Geometry: final body of the model. Coordinates: model frame, mm. Give positions to 0.01 mm unless a question says otherwise; leave off trailing zeros. Write each loop counter-clockwise with the first axis right and the second up, starting at its lowest first coordinate (ties: lowest second). Pieces come first, ordered by that corner, then holes. Notation, with made-up numbers: M 45,-33 L 54,-33 A17 cw 54,-13 Z; hole C -14,87.5 d6. An arc over 180 degrees is marked long. Answer as a JSON object with one key per item and string values.
Autodesk Fusion 360 part; units mm, degrees
sketch "plate-2025-12-04T13_16_58.583Z" plane through (0, 0, 0) normal (0, 0, 1) x (1, 0, 0)
  line L0 (3.025, -21.575) -> (16.025, -21.575)
  line L1 (3.025, -35.575) -> (16.025, -35.575)
  line L2 (2.525, -22.075) -> (2.525, -35.075)
  line L3 (16.525, -22.075) -> (16.525, -35.075)
  arc A0 (3.025, -21.575) -> (2.525, -22.075) centre (3.025, -22.075) ccw
  arc A1 (16.525, -22.075) -> (16.025, -21.575) centre (16.025, -22.075) ccw
  arc A2 (2.525, -35.075) -> (3.025, -35.575) centre (3.025, -35.075) ccw
  arc A3 (16.025, -35.575) -> (16.525, -35.075) centre (16.025, -35.075) ccw
  line L4 (22.075, -21.575) -> (35.075, -21.575)
  line L5 (22.075, -35.575) -> (35.075, -35.575)
  line L6 (21.575, -22.075) -> (21.575, -35.075)
  line L7 (35.575, -22.075) -> (35.575, -35.075)
  arc A4 (22.075, -21.575) -> (21.575, -22.075) centre (22.075, -22.075) ccw
  arc A5 (35.575, -22.075) -> (35.075, -21.575) centre (35.075, -22.075) ccw
  arc A6 (21.575, -35.075) -> (22.075, -35.575) centre (22.075, -35.075) ccw
  arc A7 (35.075, -35.575) -> (35.575, -35.075) centre (35.075, -35.075) ccw
  line L8 (3.025, -40.625) -> (16.025, -40.625)
  line L9 (3.025, -54.625) -> (16.025, -54.625)
  line L10 (2.525, -41.125) -> (2.525, -54.125)
  line L11 (16.525, -41.125) -> (16.525, -54.125)
  arc A8 (3.025, -40.625) -> (2.525, -41.125) centre (3.025, -41.125) ccw
  arc A9 (16.525, -41.125) -> (16.025, -40.625) centre (16.025, -41.125) ccw
  arc A10 (2.525, -54.125) -> (3.025, -54.625) centre (3.025, -54.125) ccw
  arc A11 (16.025, -54.625) -> (16.525, -54.125) centre (16.025, -54.125) ccw
  line L12 (22.075, -40.625) -> (35.075, -40.625)
  line L13 (22.075, -54.625) -> (35.075, -54.625)
  line L14 (21.575, -41.125) -> (21.575, -54.125)
  line L15 (35.575, -41.125) -> (35.575, -54.125)
  arc A12 (22.075, -40.625) -> (21.575, -41.125) centre (22.075, -41.125) ccw
  arc A13 (35.575, -41.125) -> (35.075, -40.625) centre (35.075, -41.125) ccw
  arc A14 (21.575, -54.125) -> (22.075, -54.625) centre (22.075, -54.125) ccw
  arc A15 (35.075, -54.625) -> (35.575, -54.125) centre (35.075, -54.125) ccw
  line L16 (0, -57.15) -> (38.1, -57.15)
  line L17 (0, -19.05) -> (38.1, -19.05)
  line L18 (0, -57.15) -> (0, -19.05)
  line L19 (38.1, -57.15) -> (38.1, -19.05)
  line L20 (-17.994, 26.134) -> (60.006, 26.134)
  line L21 (60.006, 26.134) -> (60.006, -68.197)
  line L22 (60.006, -68.197) -> (-17.994, -68.197)
  line L23 (-17.994, -68.197) -> (-17.994, 26.134)
  line L24 (6.604, 26.134) -> (25.104, 26.134)
  line L25 (25.104, 26.134) -> (25.104, -4.866)
  line L26 (25.104, -4.866) -> (6.604, -4.866)
  line L27 (6.604, -4.866) -> (6.604, 26.134)
  circle A16 centre (-12.994, 21.134) radius 1.7
  circle A17 centre (55.006, 21.134) radius 1.7
  circle A18 centre (-12.994, -63.197) radius 1.7
  circle A19 centre (55.006, -63.197) radius 1.7
  dimension "d1" = 78
  dimension "d2" = 94.331
  dimension "d4" = 20.519
  dimension "d5" = 13.572
  dimension "d6" = 18.5
  dimension "d7" = 31
  dimension "d8" = 24.598
  dimension "d9" = 3.4
  dimension "d10" = 5
  dimension "d11" = 5
  dimension "d12" = 3.4
  dimension "d13" = 5
  dimension "d14" = 5
  dimension "d15" = 3.4
  dimension "d16" = 5
  dimension "d17" = 5
  dimension "d18" = 3.4
  dimension "d19" = 5
  dimension "d20" = 5
extrude "Extrude1" add sketch "plate-2025-12-04T13_16_58.583Z" along normal blind 1.5 contours L16 L17 L18 L19 | L20 L21 L22 L23 L25 L26 L27
fillet "Fillet1" radius 5.75 1 edges at (60.006, -68.197, 0.75)
fillet "Fillet2" radius 5.75 1 edges at (-17.994, -68.197, 0.75)
fillet "Fillet3" radius 5.75 1 edges at (60.006, 26.134, 0.75)
fillet "Fillet4" radius 5.75 1 edges at (-17.994, 26.134, 0.75)
equation "d5 = 9.5 mm + 4.072 mm"
equation "d8 = 18.848 mm + 5.75 mm"
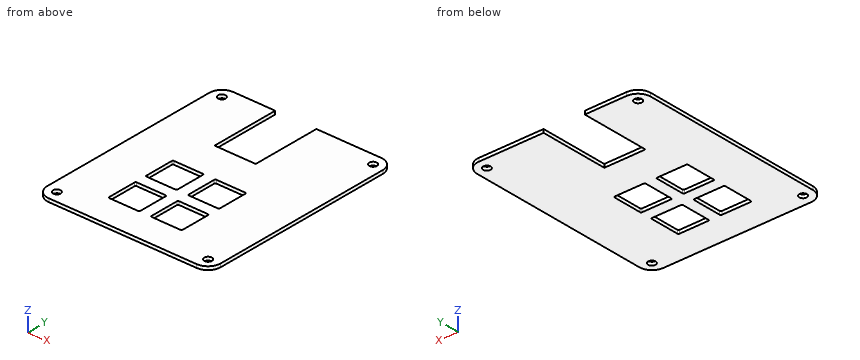
1) Cut plane D-D on z = 1.1. Give the number of separate pieces and of enclosed holes in the cut face, and give its area (3 significant figures).
Geometry check:
{"separate pieces": "1", "enclosed holes": "8", "area": "5,940 mm2"}
2) Cut plane C-C on y = -53. Return loops of the section in (x, z) (3 decimals), and give its area (3 significant figures).
Geometry check:
{"outline": "M -17.994,0 L 2.525,0 L 2.525,1.5 L -17.994,1.5 Z; M 16.525,0 L 21.575,0 L 21.575,1.5 L 16.525,1.5 Z; M 35.575,0 L 60.006,0 L 60.006,1.5 L 35.575,1.5 Z", "area": "75.0 mm2"}
3) Cut plane A-A on y = -2. Return loops of the section in (x, z).
Geometry check:
{"outline": "M -17.99,0 L 6.6,0 L 6.6,1.5 L -17.99,1.5 Z; M 25.1,0 L 60.01,0 L 60.01,1.5 L 25.1,1.5 Z"}
4) Cut plane B-B on x = 23.5. Return loops of the section in (y, z) (3 decimals), and give its area (3 significant figures).
Geometry check:
{"outline": "M -68.197,0 L -54.625,0 L -54.625,1.5 L -68.197,1.5 Z; M -40.625,0 L -35.575,0 L -35.575,1.5 L -40.625,1.5 Z; M -21.575,0 L -4.866,0 L -4.866,1.5 L -21.575,1.5 Z", "area": "53.0 mm2"}
5) Line query: line 1 (Y direction, x = 27.5, z = 1) (3 decimals); line 2 (X direction, y = -23, z = 1.3) (3 decimals); line 3 (Y direction, x = 12.5, z = 0.65) (3 decimals). Output: solid intervals per line, ascending. Write a range as from..to.
Geometry check:
{"line 1": "y = -68.197..-54.625, -40.625..-35.575, -21.575..26.134", "line 2": "x = -17.994..2.525, 16.525..21.575, 35.575..60.006", "line 3": "y = -68.197..-54.625, -40.625..-35.575, -21.575..-4.866"}
